Model file for the job. Use its own axes, mm. A direction names the side the tool comes from. Round coordinates to 2 decimals unless told otherwise and drop trailing zeros. Order: outer loops, then holes, each group sorted by start corner. A loop starts at its lowest first (then second) coordinate and runs counter-clockwise, first axis right, second up. Notation, with made-up numbers: (48.5, 33.25) - (105.5, 33.25) arc R7 cw to (105.5, 38.25) - close; hole circle Ø7 at (52, -36). An arc over 180 degrees is marked (long way). Put each result on its own line as item: value. Start each with the question number.
Item 1: Probe probe 1 along Z at (x, y) = (4, 6.5); probe 2 along Z at (x, y) = (13.5, 23); probe 3 along X at (y, z) = (5.5, -18.85). List the from-to ranges inside material, lowest first.
Item 2: Saw through at A-A on y = -2.5. List the corners of the cut face in (x, z).
Item 3: Saw through at D-D on z = -0.5. List the corners of the cut face in (x, y).
Item 4: Saw through at B-B on y = 15.5. List the corners of the cut face in (x, z).
Item 5: Pin check, flat tips, straight feed: pin 1 Ø8.5 at (x, y) = (7, 19.5) entering from -Z; pin 2 Ø2.5 at (x, y) = (10.76, 5.5) entering from -Z; pin 3 Ø2 at (x, z) = (1, 6.5) entering from -Y; pin 4 Ø10 at (x, z) = (3.5, -9.5) entering from +Y. Stop position of each tip, or through.
Item 6: Which spindle directions (+Z, -Z, +X, -X, +Y, -Y) get a long thin tool onto all of the face, cutting with end or side? Do faces 1 (the face through (6, 3, -15)), 2 (the face through (6, 2, -21.135)), 3 (the face through (6, 18, -7)), 4 (the face through (5.88, 29.7, 23.88)). Say none if no direction does.
Item 7: Mould opens along Z. For faces 5 (the face through (5.882, 3.285, 23.864)), 6 (the face through (6, 9, -20)), 7 (the face through (5.64, 32.7, -8.85)) say: pulls with the +Z half, pulls with the -Z half, needs draft (parallel to the pull), parting line crosses it, or undercut.
Item 8: Saw through at C-C on y = 25. List the corners of the cut face in (x, z).
```python
from build123d import *

# Parameters (mm, degrees)
SKETCH1_W           = 17
SKETCH1_H           = 47
SKETCH1_R           = 3.5
BOSS_EXTRUDE1_DEPTH = 3
SKETCH2_W           = 17
SKETCH2_H           = 8
SKETCH2_H_2         = 1.7
BOSS_EXTRUDE2_DEPTH = 27
SKETCH3_W           = 17
SKETCH3_H           = 35
BOSS_EXTRUDE3_DEPTH = 3
SKETCH4_R           = 3.5
CUT_EXTRUDE1_DEPTH  = 3
SKETCH5_R           = 1.5
SKETCH5_R_2         = 1.331036909
CUT_EXTRUDE2_DEPTH  = 15
SKETCH7_W           = 12.5
SKETCH7_H           = 23
CUT_EXTRUDE3_DEPTH  = 30
SKETCH8_W           = 17
SKETCH8_H           = 15
SKETCH8_R           = 1.5
BOSS_EXTRUDE4_DEPTH = 3
SKETCH9_W           = 2.25
SKETCH9_H           = 22.972634834
CUT_EXTRUDE4_DEPTH  = 30
FILLET8_R           = 3
FILLET9_R           = 3
FILLET10_R          = 3
FILLET11_R          = 3
FILLET12_R          = 3
FILLET13_START      = -2.737421384
FILLET13_DEPTH      = 17
FILLET14_START      = -2.737421384
FILLET14_DEPTH      = 17
FILLET15_R          = 1
FILLET16_R          = 1
FILLET17_R          = 1


with BuildPart() as part:
    # Sketch1 → Boss-Extrude1 (new body)
    with BuildSketch(Plane(origin=(0, 0, 0), x_dir=(1, 0, 0), z_dir=(0, 1, 0))):
        with Locations((5.762578616, -2.364779874)):
            Rectangle(SKETCH1_W, SKETCH1_H)
        with Locations(Location((5.762578616, -13.864779874, 0), (0, 0, 270))):
            Circle(SKETCH1_R, mode=Mode.SUBTRACT)
    extrude(amount=BOSS_EXTRUDE1_DEPTH)

    # Sketch2 → Boss-Extrude2 (add)
    with BuildSketch(Plane(origin=(0, 3, 0), x_dir=(1, 0, 0), z_dir=(0, 1, 0))):
        with Locations((5.762578616, 5.135220126)):
            Rectangle(SKETCH2_W, SKETCH2_H)
        with Locations((5.762578616, -25.014779874)):
            Rectangle(SKETCH2_W, SKETCH2_H_2)
    extrude(amount=BOSS_EXTRUDE2_DEPTH)

    # Sketch3 → Boss-Extrude3 (add)
    with BuildSketch(Plane(origin=(0, 30, 0), x_dir=(1, 0, 0), z_dir=(0, 1, 0))):
        with Locations((5.762578616, -8.364779874)):
            Rectangle(SKETCH3_W, SKETCH3_H)
    extrude(amount=BOSS_EXTRUDE3_DEPTH)

    # Sketch4 → Cut-Extrude1 (cut)
    with BuildSketch(Plane.XZ.offset(-30)):
        with Locations(Location((5.762578616, 13.864779874, 0), (0, 0, 90))):
            Circle(SKETCH4_R)
    extrude(amount=-CUT_EXTRUDE1_DEPTH, mode=Mode.SUBTRACT)

    # Sketch5 → Cut-Extrude2 (cut)
    with BuildSketch(Plane(origin=(0, 33, 0), x_dir=(1, 0, 0), z_dir=(0, 1, 0))):
        with Locations(Location((5.762578616, -20.864779874, 0), (0, 0, 270))):
            Circle(SKETCH5_R)
        with Locations(Location((5.762578616, 6.885220126, 0), (0, 0, 270))):
            Circle(SKETCH5_R_2)
    extrude(amount=-CUT_EXTRUDE2_DEPTH, mode=Mode.SUBTRACT)

    # Sketch7 → Cut-Extrude3 (cut)
    with BuildSketch(Plane(origin=(0, 33, 0), x_dir=(1, 0, 0), z_dir=(0, 1, 0))):
        with Locations((5.762578616, -6.989779874)):
            Rectangle(SKETCH7_W, SKETCH7_H)
    extrude(amount=-CUT_EXTRUDE3_DEPTH, mode=Mode.SUBTRACT)

    # Sketch8 → Boss-Extrude4 (add)
    with BuildSketch(Plane(origin=(0, 0, -21.135220126), x_dir=(-1, 0, 0), z_dir=(0, 0, -1))):
        with Locations((-5.762578616, 1.5)):
            Rectangle(SKETCH8_W, SKETCH8_H)
        with Locations((-10.762578616, 5.5)):
            Circle(SKETCH8_R, mode=Mode.SUBTRACT)
        with Locations((-0.762578616, 5.5)):
            Circle(SKETCH8_R, mode=Mode.SUBTRACT)
        with Locations((-10.762578616, -2.5)):
            Circle(SKETCH8_R, mode=Mode.SUBTRACT)
        with Locations((-0.762578616, -2.5)):
            Circle(SKETCH8_R, mode=Mode.SUBTRACT)
    extrude(amount=-BOSS_EXTRUDE4_DEPTH)

    # Sketch9 → Cut-Extrude4 (cut)
    with BuildSketch(Plane(origin=(0, 33, 0), x_dir=(1, 0, 0), z_dir=(0, 1, 0))):
        with Locations((13.137578616, -6.976097291)):
            Rectangle(SKETCH9_W, SKETCH9_H)
    extrude(amount=-CUT_EXTRUDE4_DEPTH, mode=Mode.SUBTRACT)

    # Fillet8
    fillet8_edges = [part.edges().sort_by_distance(p)[0] for p in [
        (5.762578616, 0, 25.864779874),
    ]]
    fillet(fillet8_edges, radius=FILLET8_R)

    # Fillet9
    fillet9_edges = [part.edges().sort_by_distance(p)[0] for p in [
        (5.762578616, 33, 25.864779874),
    ]]
    fillet(fillet9_edges, radius=FILLET9_R)

    # Fillet10
    fillet10_edges = [part.edges().sort_by_distance(p)[0] for p in [
        (5.762578616, 3, -9.135220126),
    ]]
    fillet(fillet10_edges, radius=FILLET10_R)

    # Fillet11
    fillet11_edges = [part.edges().sort_by_distance(p)[0] for p in [
        (6.887578616, 3, -4.510220126),
    ]]
    fillet(fillet11_edges, radius=FILLET11_R)

    # Fillet12
    fillet12_edges = [part.edges().sort_by_distance(p)[0] for p in [
        (-1.612421384, 3, -1.135220126),
    ]]
    fillet(fillet12_edges, radius=FILLET12_R)

    # Fillet13: read off the stored shape, not the designer's step
    # Fillet13 outline → Fillet13 (add)
    with BuildSketch(Plane.YZ.offset(FILLET13_START)):
        with BuildLine():
            Line((3, -18.135220126), (4, -18.135220126))
            ThreePointArc((4, -18.135220126), (3.292893219, -17.842326907), (3, -17.135220126))
            Line((3, -17.135220126), (3, -18.135220126))
        make_face()
    extrude(amount=FILLET13_DEPTH)

    # Fillet14: read off the stored shape, not the designer's step
    # Fillet14 outline → Fillet14 (add)
    with BuildSketch(Plane.YZ.offset(FILLET14_START)):
        with BuildLine():
            ThreePointArc((0, -17.135220126), (-0.292893219, -17.842326907), (-1, -18.135220126))
            Line((-1, -18.135220126), (0, -18.135220126))
            Line((0, -18.135220126), (0, -17.135220126))
        make_face()
    extrude(amount=FILLET14_DEPTH)

    # Fillet15
    fillet15_edges = [part.edges().sort_by_distance(p)[0] for p in [
        (5.762578616, 3, 24.164779874),
    ]]
    fillet(fillet15_edges, radius=FILLET15_R)

    # Fillet16
    fillet16_edges = [part.edges().sort_by_distance(p)[0] for p in [
        (5.762578616, 30, 24.164779874),
    ]]
    fillet(fillet16_edges, radius=FILLET16_R)

    # Fillet17
    # the kernel refuses this fillet: 1 mm, written as the material it takes off along each edge
    with BuildSketch(Plane(origin=(-5.237421384, 33, -9.135220126), x_dir=(0, -1, 0), z_dir=(1, 0, 0))) as fillet17_piece_1:
        with BuildLine():
            CenterArc((FILLET17_R, -FILLET17_R), FILLET17_R, 90, 90)
            Line((0, -FILLET17_R), (0, 0))
            Line((0, 0), (FILLET17_R, 0))
        make_face()
    extrude(amount=22, mode=Mode.SUBTRACT)


solid = part.part
```
Results found:
1. probe 1: z = -21.14 to -18.14, -9.14 to -4.51, 24.16 to 25.86
1. probe 2: z = -9.14 to -4.51, 24.16 to 25.86
1. probe 3: x = -2.74 to -0.74, 2.26 to 9.26, 12.26 to 14.26
2. outline: (-2.74, -21.14) - (-0.74, -21.14) - (-0.74, -18.14) - (-2.74, -18.14) - close; (2.26, -21.14) - (9.26, -21.14) - (9.26, -18.14) - (2.26, -18.14) - close; (12.26, -21.14) - (14.26, -21.14) - (14.26, -18.14) - (12.26, -18.14) - close
3. outline: (-2.74, 0) - (14.26, 0) - (14.26, 3) - (-0.49, 3) - (-0.49, 4.15) - (-2.74, 4.15) - close; (-2.74, 30) - (-0.49, 30) - (-0.49, 33) - (-2.74, 33) - close
4. outline: (-2.74, -9.14) - (14.26, -9.14) - (14.26, -4.51) - (-0.49, -4.51) - (-0.49, -1.14) - (-2.74, -1.14) - close; (-2.74, 24.16) - (14.26, 24.16) - (14.26, 25.86) - (-2.74, 25.86) - close
5. pin 1: stops at z = -9.14
5. pin 2: stops at z = -9.7
5. pin 3: stops at y = 0
5. pin 4: stops at y = 33
6. face 1: +X, -X, +Y
6. face 2: -Z, +X, -X, +Y, -Y
6. face 3: +Y
6. face 4: +X, -X
7. face 5: undercut
7. face 6: needs draft
7. face 7: pulls with the -Z half
8. outline: (-2.74, -9.14) - (14.26, -9.14) - (14.26, -4.51) - (-0.49, -4.51) - (-0.49, -1.14) - (-2.74, -1.14) - close; (-2.74, 24.16) - (14.26, 24.16) - (14.26, 25.86) - (-2.74, 25.86) - close; hole circle Ø2.66 at (5.76, -6.89)
